Read the model definition and answer for the solid it produces. Units are mm, in the model's axes. Face numbers are marked on the shaded views. A direction names the side the tool comes from. Coordinates: 2 decimals unless noted, no trailing zeros. Order: outer loops, then holes, each group sorted by start corner. A loop starts at its lowest first (then second) coordinate and runs counter-clockwise, first axis right, second up.
```python
from build123d import *

# Parameters (mm, degrees)
F0_R          = 53
F1_DEPTH      = 18
F2_R          = 53
F2_R_2        = 50
F3_DEPTH      = 68
F3_DEPTH_BACK = 80
F4_R          = 93
F4_R_2        = 53
F5_DEPTH      = 18
F6_R          = 93
F6_R_2        = 53
F7_DEPTH      = 18
F8_R          = 5


with BuildPart() as f1:
    # F0 (on Front) → F1 (new body)
    with BuildSketch(Plane.XZ):
        with BuildLine():
            Line((0, 333.882748), (261, 333.882748))
            Line((261, 333.882748), (261, 431))
            ThreePointArc((261, 431), (275.644661, 466.355339), (311, 481))
            Line((311, 481), (386, 481))
            ThreePointArc((386, 481), (421.355339, 495.644661), (436, 531))
            Line((436, 531), (436, 742.312182))
            ThreePointArc((436, 742.312182), (421.355339, 777.667521), (386, 792.312182))
            Line((386, 792.312182), (382.797237, 792.312182))
            ThreePointArc((382.797237, 792.312182), (361.988427, 796.847982), (344.955002, 809.632443))
            ThreePointArc((344.955002, 809.632443), (267, 845.312182), (189.044998, 809.632443))
            ThreePointArc((189.044998, 809.632443), (172.011573, 796.847982), (151.202763, 792.312182))
            Line((151.202763, 792.312182), (120, 792.312182))
            Line((120, 792.312182), (120, 692.312182))
            Line((120, 692.312182), (102, 692.312182))
            Line((102, 692.312182), (102, 792.312182))
            Line((102, 792.312182), (32, 792.312182))
            ThreePointArc((32, 792.312182), (-3.355339, 777.667521), (-18, 742.312182))
            Line((-18, 742.312182), (-18, 741.883182))
            Line((-18, 741.883182), (0, 741.883182))
            Line((0, 741.883182), (0, 333.882748))
        make_face()
        with Locations((267, 742.312182)):
            Circle(F0_R, mode=Mode.SUBTRACT)
    extrude(amount=F1_DEPTH)

    # F2 (on face) → F3 (join, two sides)
    with BuildSketch(Plane(origin=(0, 0, 0), x_dir=(-1, 0, 0), z_dir=(0, 1, 0))) as f3_sk:
        with Locations((-267, 742.312182)):
            Circle(F2_R)
        with Locations((-267, 742.312182)):
            Circle(F2_R_2, mode=Mode.SUBTRACT)
    extrude(amount=F3_DEPTH)
    extrude(f3_sk.sketch, amount=-F3_DEPTH_BACK)

    # F4 (on face) → F5 (join)
    with BuildSketch(Plane(origin=(0, 0, 0), x_dir=(-1, 0, 0), z_dir=(0, 1, 0))):
        with Locations((-267, 742.312182)):
            Circle(F4_R)
        with Locations((-267, 742.312182)):
            Circle(F4_R_2, mode=Mode.SUBTRACT)
    extrude(amount=F5_DEPTH)

    # F6 (on face) → F7 (join)
    with BuildSketch(Plane.XZ.offset(18)):
        with Locations((267, 742.312182)):
            Circle(F6_R)
        with Locations((267, 742.312182)):
            Circle(F6_R_2, mode=Mode.SUBTRACT)
    extrude(amount=F7_DEPTH)

    # F8
    f8_edges = [f1.edges().sort_by_distance(p)[0] for p in [
        (360, 18, 742.312182),
        (174, -36, 742.312182),
    ]]
    fillet(f8_edges, radius=F8_R)


solid = f1.part
```
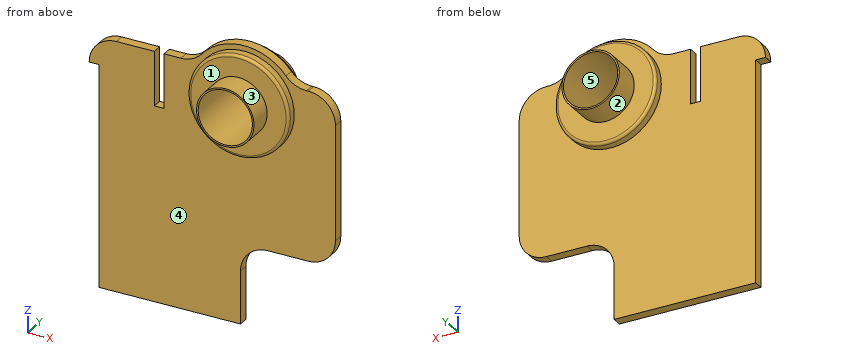
1) Determine the mould class of the marked faces 3, 4 and 5 for opening direction X: pulls with the +X half, pulls with the -X half, needs draft (parallel to the pull), parting line crosses it, or undercut.
A:
face 3: parting line crosses it
face 4: needs draft
face 5: undercut
2) A cutting plane is placed at B-B, the plane x = 267. Determine the outline of the cut face in (y, z), and give its area (3 significant figures).
A:
outline: (-80, 689.31) - (-36, 689.31) - (-36, 654.31) arc R5 ccw to (-31, 649.31) - (-18, 649.31) - (-18, 454.75) - (0, 454.75) - (0, 649.31) - (13, 649.31) arc R5 ccw to (18, 654.31) - (18, 689.31) - (68, 689.31) - (68, 692.31) - (-80, 692.31) - close; (-80, 792.31) - (68, 792.31) - (68, 795.31) - (18, 795.31) - (18, 830.31) arc R5 ccw to (13, 835.31) - (0, 835.31) - (0, 845.31) - (-18, 845.31) - (-18, 835.31) - (-31, 835.31) arc R5 ccw to (-36, 830.31) - (-36, 795.31) - (-80, 795.31) - close
area: 8,870 mm2
3) Which of the six approach directions +Z, -Z, +X, -X, +Y, -Y give full straight-line access (tool end or side, diameter ignored) to the marked faces 1 and 2?
A:
face 1: -Y
face 2: +Y
4) Flat-ended cylindrical pins translate along their axes: pin 1 Ø5.5 at (x, y) = (345, -7) entering from -Z; pin 2 Ø1.5 at (y, z) = (-49, 752.5) entering from -X; pin 3 Ø1.5 at (y, z) = (-0.5, 402) entering from +X. Find the tip coordinate at first contact, or state that the pin passes through.
A:
pin 1: stops at z = 481
pin 2: stops at x = 214.85
pin 3: stops at x = 261
5) A cutting plane is placed at C-C, the plane z = 581.5. Determine the outline of the cut face in (x, y).
A:
outline: (0, -18) - (436, -18) - (436, 0) - (0, 0) - close
6) A cutting plane is placed at D-D, the plane x = 113.5. Determine the outline of the cut face in (y, z), and give its area (3 significant figures).
A:
outline: (-18, 333.88) - (0, 333.88) - (0, 692.31) - (-18, 692.31) - close
area: 6,450 mm2
7) Straight lines are drawn through the part: line 1 (Z direction, x = 264.5, y = -67.5); line 2 (Z direction, x = 267, y = 24); line 3 (X direction, y = -11, z = 707). For each, find the intervals that lie inside material, in ascending order.
A:
line 1: z = 689.37 to 692.37, 792.25 to 795.25
line 2: z = 689.31 to 692.31, 792.31 to 795.31
line 3: x = 0 to 102, 120 to 231.6, 302.4 to 436
8) A cutting plane is placed at A-A, the plane y = -55.5. Determine the outline of the cut face in (x, z), and give its area (3 significant figures).
A:
outline: circle Ø106 at (267, 742.31); hole circle Ø100 at (267, 742.31)
area: 971 mm2
